Work out the finished part from the listing and answer in its coordinate system (mm). Give positions to 0.01 mm unless a question says otherwise; leave off trailing zeros. Loops run counter-clockwise (first coordinate to the right, second up) from the corner with the lowest first, then second, coordinate; pieces in that order, holes last. Notation, with made-up numbers: (18.5, 62.25) - (42.5, 62.25) arc R32 cw to (42.5, 90.25) - close; hole circle Ø10 at (67, -14.75). An arc over 180 degrees is marked (long way). One line per question, with ' | ' between items.
from build123d import *

# Parameters (mm, degrees)
SKIZZE2_W                       = 70
SKIZZE2_H                       = 70
AUFSATZ_LINEAR_AUSTRAGEN2_DEPTH = 10
SKIZZE5_R                       = 2.55
SCHNITT_LINEAR_AUSTRAGEN1_DEPTH = 10
FASE2_SIZE                      = 50
FASE2_SIZE2                     = 28.867513459
FASE3_SIZE                      = 50
FASE3_SIZE2                     = 28.867513459


with BuildPart() as part:
    # Skizze2 → Aufsatz-Linear austragen2 (new body)
    with BuildSketch(Plane.XY):
        with Locations((35, 35)):
            Rectangle(SKIZZE2_W, SKIZZE2_H)
    extrude(amount=AUFSATZ_LINEAR_AUSTRAGEN2_DEPTH)

    # Skizze5 → Schnitt-Linear austragen1 (cut)
    with BuildSketch(Plane.XY.offset(10)):
        with Locations((35, 63)):
            Circle(SKIZZE5_R)
        with Locations((59.248711306, 21)):
            Circle(SKIZZE5_R)
        with Locations((10.751288694, 21)):
            Circle(SKIZZE5_R)
    extrude(amount=-SCHNITT_LINEAR_AUSTRAGEN1_DEPTH, mode=Mode.SUBTRACT)

    # Fase2
    fase2_edges = [part.edges().sort_by_distance(p)[0] for p in [
        (70, 70, 5),
    ]]
    fase2_side = [part.faces().sort_by_distance(p)[0] for p in [
        (70, 35, 5),
    ]]
    chamfer(fase2_edges, length=FASE2_SIZE, length2=FASE2_SIZE2, reference=fase2_side[0])

    # Fase3
    fase3_edges = [part.edges().sort_by_distance(p)[0] for p in [
        (0, 70, 5),
    ]]
    fase3_side = [part.faces().sort_by_distance(p)[0] for p in [
        (0, 35, 5),
    ]]
    chamfer(fase3_edges, length=FASE3_SIZE, length2=FASE3_SIZE2, reference=fase3_side[0])


solid = part.part
1. Find section A-A on x = 35. Write down the section's boundary in (y, z).
Evaluation:
outline: (0, 0) - (60.45, 0) - (60.45, 10) - (0, 10) - close; (65.55, 0) - (70, 0) - (70, 10) - (65.55, 10) - close
2. Find section B-B on z = 7.5. Write down the section's boundary in (x, y).
Evaluation:
outline: (0, 0) - (70, 0) - (70, 20) - (41.13, 70) - (28.87, 70) - (0, 20) - close; hole circle Ø5.1 at (10.75, 21); hole circle Ø5.1 at (35, 63); hole circle Ø5.1 at (59.25, 21)
3. Find section C-C on y = 63. Write down the section's boundary in (x, z), then the cut area to 3 significant figures.
Evaluation:
outline: (24.83, 0) - (32.45, 0) - (32.45, 10) - (24.83, 10) - close; (37.55, 0) - (45.17, 0) - (45.17, 10) - (37.55, 10) - close | area: 152 mm2
4. Determine the mould class of faces 1 (the cylindrical face through (61.68, 21.77, 5.07)), 2 (the flat face through (70, 10, 5)), 3 (the flat face through (14.636, 45.35, 4.93)), 4 (the flat face through (35, 28, 10)) for opening direction X: +X half, -X half, draft (parallel to the pull), parting line (faces both ways), or undercut.
Evaluation:
face 1: undercut | face 2: +X half | face 3: -X half | face 4: draft
5. Consider L1, parallel to Y at x = 35, z = 6; L2, parallel to Y at x = 12.5, z = 4.5; L3, parallel to Y at x = 6.5, z = 3. Determine where each line is inside the solid, lowest interval first.
Evaluation:
L1: 0 to 60.45, 65.55 to 70 | L2: 0 to 19.14, 22.86 to 41.65 | L3: 0 to 31.26
6. Find section D-D on y = 21. Write down the section's boundary in (x, z).
Evaluation:
outline: (0.58, 0) - (8.2, 0) - (8.2, 10) - (0.58, 10) - close; (13.3, 0) - (56.7, 0) - (56.7, 10) - (13.3, 10) - close; (61.8, 0) - (69.42, 0) - (69.42, 10) - (61.8, 10) - close
